```python
from build123d import *

# Parameters (mm, degrees)
BOSS_EXTRUDE2_DEPTH   = 11
BOSS_EXTRUDE2_2_DEPTH = 11
BOSS_EXTRUDE3_START   = 11
BOSS_EXTRUDE3_DEPTH   = 1
FILLET2_R             = 10
FILLET1_R             = 2
BOSS_EXTRUDE4_DEPTH   = 11
TUBE_HOLES_DEPTH      = 10
POT_INSERT_DEPTH      = 2.5
POT_START             = -2.5
SKETCH13_R            = 2.75
POT_HOLE_DEPTH        = 1.5
SKETCH7_R             = 0.8
SCREW_HOLES_DEPTH     = 12
SCREW_START           = 11
SKETCH12_R            = 1.25
SCREW_HEADS_DEPTH     = 3


with BuildPart() as part:
    # Sketch3 → Boss-Extrude2 (new body)
    with BuildSketch(Plane(origin=(0, 0, 0), x_dir=(1, 0, 0), z_dir=(0, 1, 0))):
        Polygon((-2.631461599, 29.291458176), (-6.631461599, 29.291458176), (-6.631461599, 5.791458176), (7.368538401, -8.208541824), (35.368538401, -8.208541824), (35.368538401, 15.791458176), (41.368538401, 21.791458176), (41.368538401, 29.291458179), (35.368538401, 29.291458179), (35.368538401, 33.291458176), (31.368538401, 33.291458176), (31.368538401, 29.291458176), (34.368538401, 29.291458176), (34.368538401, 28.291458176), (39.368538401, 28.291458176), (39.368538401, 22.619885301), (35.040111276, 18.291458176), (31.368538401, 18.291458176), (31.368538401, 11.791458176), (34.368538401, 14.791458176), (34.368538401, 5.306176806), (31.368538401, 2.306176806), (31.368538401, -0.708541824), (34.368538401, -0.708541824), (34.368538401, -4.208541824), (31.368538401, -4.208541824), (31.368538401, -7.208541824), (12.02539265, -7.208541824), (-2.631461599, 7.448312426), (-2.631461599, 12.291458176), (-5.631461599, 12.291458176), (-5.631461599, 25.291458176), (-2.631461599, 25.291458176), align=None)
    extrude(amount=BOSS_EXTRUDE2_DEPTH)



with BuildPart() as body_2:
    # Sketch3 → Boss-Extrude2 2 (new body)
    with BuildSketch(Plane(origin=(0, 0, 0), x_dir=(1, 0, 0), z_dir=(0, 1, 0))):
        Polygon((9.368538401, 29.291458176), (15.368538401, 29.291458176), (15.368538401, 33.291458176), (19.368538401, 33.291458176), (19.368538401, 28.291458176), (9.368538401, 28.291458176), align=None)
    extrude(amount=BOSS_EXTRUDE2_2_DEPTH)


with BuildPart() as part_1:
    add(part.part)

    add(body_2.part)  # Boss-Extrude3 merges body 2
    # Sketch5 → Boss-Extrude3 (add)
    with BuildSketch(Plane(origin=(0, 0, 0), x_dir=(1, 0, 0), z_dir=(0, 1, 0)).offset(BOSS_EXTRUDE3_START)):
        Polygon((-6.631461599, 29.291458176), (15.368538401, 29.291458176), (15.368538401, 33.291458176), (35.368538401, 33.291458176), (35.368538401, 29.291458179), (41.368538401, 29.291458179), (41.368538401, 21.791458176), (35.368538401, 15.791458176), (35.368538401, -8.208541824), (7.368538401, -8.208541824), (-6.631461599, 5.791458176), align=None)
    extrude(amount=-BOSS_EXTRUDE3_DEPTH)

    # Fillet2
    fillet2_edges = [part_1.edges().sort_by_distance(p)[0] for p in [
        (41.368538401, 5.5, -21.791458176),
    ]]
    fillet(fillet2_edges, radius=FILLET2_R)

    # Fillet1
    fillet1_edges = [part_1.edges().sort_by_distance(p)[0] for p in [
        (36.904072307, 11, -17.326992082),
        (41.368538401, 11, -27.61252599),
        (35.368538401, 11, -31.291458178),
        (15.368538401, 11, -31.291458176),
        (40.607333726, 11, -22.106759476),
        (-6.631461599, 11, -17.541458176),
        (0.368538401, 11, 1.208541824),
    ]]
    fillet(fillet1_edges, radius=FILLET1_R)

    # Sketch14 → Boss-Extrude4 (add)
    with BuildSketch(Plane(origin=(0, 0, 0), x_dir=(1, 0, 0), z_dir=(0, 1, 0))):
        Polygon((31.368538401, 11.791458176), (35.368538401, 15.791458176), (35.368538401, 17.791458176), (31.368538401, 13.791458176), align=None)
    extrude(amount=BOSS_EXTRUDE4_DEPTH)

    # Sketch10 → Tube Holes (cut)
    with BuildSketch(Plane(origin=(0, 0, 0), x_dir=(1, 0, 0), z_dir=(0, 1, 0))):
        Polygon((34.368538401, 5.306176806), (35.368538401, 6.306176806), (35.368538401, 15.791458176), (34.368538401, 14.791458176), align=None)
        Polygon((10.368538401, -5.551687574), (10.368538401, -8.208541824), (31.368538401, -8.208541824), (31.368538401, -3.516153668), (17.52539265, -3.516153668), (6.918790933, 7.09044805), (2.322596855, 2.494253972), align=None)
    extrude(amount=TUBE_HOLES_DEPTH, mode=Mode.SUBTRACT)

    # Sketch9 → Pot Insert (cut)
    with BuildSketch(Plane(origin=(-0.420001711, 0, 0.420001711), x_dir=(0.707106781, 0, 0.707106781), z_dir=(-0.707106781, 0, 0.707106781))):
        Polygon((-8.284330815, 0), (-8.284330815, -1.5), (-6.784330815, -4.5), (-6.784330815, -5.5), (-2.784330815, -5.5), (1.465669185, -5.5), (1.465669185, -4.5), (6.715669185, -4.5), (6.715669185, 0), align=None)
        Polygon((-8.284330815, 1.5), (-8.284330815, 0), (6.715669185, 0), (6.715669185, 4.5), (1.465669185, 4.5), (1.465669185, 5.5), (-2.784330815, 5.5), (-6.784330815, 5.5), (-6.784330815, 4.5), align=None)
    extrude(amount=-POT_INSERT_DEPTH, mode=Mode.SUBTRACT)

    # Sketch13 → Pot Hole (cut)
    with BuildSketch(Plane(origin=(-0.420001711, 0, 0.420001711), x_dir=(0.707106781, 0, 0.707106781), z_dir=(-0.707106781, 0, 0.707106781)).offset(POT_START)):
        with Locations((-2.784330815, 0)):
            Circle(SKETCH13_R)
        Polygon((6.715669185, 0), (6.715669185, 2.5), (4.715669185, 2.5), (4.715669185, -2.5), (6.715669185, -2.5), align=None)
    extrude(amount=-POT_HOLE_DEPTH, mode=Mode.SUBTRACT)

    # Sketch7 → Screw Holes (cut, through all)
    with BuildSketch(Plane(origin=(0, 0, 0), x_dir=(1, 0, 0), z_dir=(0, 1, 0))):
        with Locations((-4.631461599, 27.291458176)):
            Circle(SKETCH7_R)
        with Locations((17.368538401, 31.291458176)):
            Circle(SKETCH7_R)
        with Locations((33.368538401, 31.291458176)):
            Circle(SKETCH7_R)
        with Locations((-4.631461599, 10.291458176)):
            Circle(SKETCH7_R)
        with Locations((33.368538401, 16.291458176)):
            Circle(SKETCH7_R)
        with Locations((8.282751963, -6.294328261)):
            Circle(SKETCH7_R)
        with Locations((33.368538401, 1.291458176)):
            Circle(SKETCH7_R)
        with Locations((33.368538401, -6.208541824)):
            Circle(SKETCH7_R)
    extrude(amount=SCREW_HOLES_DEPTH, mode=Mode.SUBTRACT)

    # Sketch12 → Screw Heads (cut)
    with BuildSketch(Plane(origin=(0, 0, 0), x_dir=(1, 0, 0), z_dir=(0, 1, 0)).offset(SCREW_START)):
        with Locations((-4.631461599, 27.291458176)):
            Circle(SKETCH12_R)
        with Locations((17.368538401, 31.291458176)):
            Circle(SKETCH12_R)
        with Locations((33.368538401, 31.291458176)):
            Circle(SKETCH12_R)
        with Locations((-4.631461599, 10.291458176)):
            Circle(SKETCH12_R)
        with Locations((33.368538401, 16.291458176)):
            Circle(SKETCH12_R)
        with Locations((8.282751963, -6.294328261)):
            Circle(SKETCH12_R)
        with Locations((33.368538401, 1.291458176)):
            Circle(SKETCH12_R)
        with Locations((33.368538401, -6.208541824)):
            Circle(SKETCH12_R)
    extrude(amount=-SCREW_HEADS_DEPTH, mode=Mode.SUBTRACT)


solid = part_1.part
```
Check sheet for the modelled part. Datum: model origin and axes. Units: mm. A direction names the side the tool comes from. Round coordinates to 2 decimals unless told otherwise and drop trailing zeros. Order: outer loops, then holes, each group sorted by start corner. A loop starts at its lowest first (then second) coordinate and runs counter-clockwise, first axis right, second up. Notation, with made-up numbers: (25.5, 12) - (74.5, 12) arc R24 cw to (74.5, 41) - close; hole circle Ø1 at (14.5, -25.75). An arc over 180 degrees is marked (long way). Write item = value, one per line.
Q1. Thickness scan on line 1 along X through (y, z) = (2, -2); line 2 along X through (y, z) = (6.5, -13); line 3 along Y through (x, z) = (28.5, -14). Record the ranges inside material, lowest first.
Computed:
line_1 = 0.73 to 2.82, 31.37 to 33, 33.74 to 35.37
line_2 = -6.63 to -5.63, 31.37 to 32.58
line_3 = 10 to 11
Q2. Section check B-B (x = 26.5). Record the boundary of the cut face in (y, z).
Computed:
outline = (10, -33.29) - (11, -33.29) - (11, 8.21) - (10, 8.21) - close
Q3. Draft check along Z on faces 1 (the face through (4, 0, 0)), 2 (the face through (33, 5, 4.209)), 3 (the face through (37, 5, -28.291)). Enter one of: pulls with the +Z half, pulls with the -Z half, needs draft (parallel to the pull), parting line crosses it, or undercut.
Computed:
face_1 = needs draft
face_2 = undercut
face_3 = undercut
Q4. Section check A-A (y = 6.75). State how many separate pieces and enclosed holes the cut face has, and give its area (3 significant figures).
Computed:
separate_pieces = 4
enclosed_holes = 8
area = 247 mm^2
Q5. Tool access check on faces 4 (the face through (34.99, 10.17, -31.32)), 5 (the face through (-2.631, 5, -27)), 6 (the face through (34.369, 5, -29)), 7 (the face through (-3.44, 9.52, -10.67)), 8 (the face through (31.369, 5, 6)). Record the directions out of +Z, -Z, +X, -X, +Y, -Y that give a thin tool (end or side, any length) a straight path to the whole face; none if there is none.
Computed:
face_4 = -Z, +X, +Y
face_5 = -Z, -Y
face_6 = -Y
face_7 = +Y
face_8 = +Z, -Z, -Y
Q6. Go/stop test with flat-tipped pins: pin 1 (1.4 mm diameter, centred on x = 33.37, z = -31.29, fed in from -Y); pin 2 (6 mm diameter, centred on x = 13.5, z = -10, fed in from -Y); pin 3 (2 mm diameter, centred on y = 5, z = -31, fed in from -X); pin 4 (6 mm diameter, centred on y = 6, z = -7, fed in from +X). Record where each tip stops, or that it passes through.
Computed:
pin_1 = through
pin_2 = 10
pin_3 = 15.37
pin_4 = 35.37
